Autodesk Inventor part; units mm, degrees
ref_plane "YZ Plane" through (0, 0, 0) normal (1, 0, 0) x (0, 1, 0)
ref_plane "XZ Plane" through (0, 0, 0) normal (0, 1, 0) x (-1, 0, 0)
ref_plane "XY Plane" through (0, 0, 0) normal (0, 0, 1) x (1, 0, 0)
sketch "Szkic1" plane through (0, 0, 0) normal (0, 1, 0) x (-1, 0, 0)
  line L0 (0, 10.6544) -> (0, -29.3456)
  line L1 (0, -29.3456) -> (40, -29.3456)
  line L2 (0, 10.6544) -> (40, 10.6544)
  arc A0 (40, -29.3456) -> (40, 10.6544) centre (40, -9.3456) ccw
  point P0 (0, 0)
  dimension "d0" = 40
  dimension "d1" = 40
extrude "Wyciągnięcie proste1" add sketch "Szkic1" along normal blind 9.5
sketch "Szkic2" plane through (0, 9.5, 0) normal (0, 1, 0) x (1, 0, 0)
  line L0 (-40, -10.6544) -> (0, -10.6544)
  line L1 (0.0007, -10.6544) -> (-40, -10.6544)
  arc A0 (-40, 29.3456) -> (-40, -10.6544) centre (-40, 9.3456) ccw
  circle A1 centre (-40, 9.3456) radius 15
  circle A2 centre (-40, 9.3456) radius 10
  point P0 (0, 0)
  dimension "d4" = 30
  dimension "d5" = 20
extrude "Wyciągnięcie proste2" add sketch "Szkic2" along normal blind 3
fillet "Zaokrąglenie1" radius 3 1 edges at (-55, 9.5, -9.3456)
sketch "Szkic3" plane through (0, 0, 0) normal (0, -1, 0) x (1, 0, 0)
  line L0 (0, 10.6544) -> (0, -29.3456)
  line L1 (0, -29.3456) -> (-16, -29.3456)
  line L2 (0, -29.3456) -> (-40, -29.3456)
  line L3 (-16, -29.3456) -> (-16, 10.6544)
  line L4 (-40, 10.6544) -> (0, 10.6544)
  line L5 (-16, 10.6544) -> (0, 10.6544)
  line L6 (0, 10.6544) -> (0, -29.3456)
  point P0 (0, 0)
  dimension "d9" = 16
  dimension "d10" = 40
extrude "Wyciągnięcie proste3" add sketch "Szkic3" along normal blind 12.5
sketch "Szkic4" plane through (-40, 9.5, -9.3456) normal (0, 1, 0) x (1, 0, 0)
  point P0 (40, -9.3456)
mirror "Odbij1" about plane through (-8, -12.5, -9.3456) normal (0, -1, 0)
sketch "Szkic7" plane through (0, 9.5, 10.6544) normal (1, 0, 0) x (0, 0, -1)
  point P0 (10.6544, -9.5)
sketch "Szkic8" plane through (0, 9.5, 10.6544) normal (1, 0, 0) x (0, 0, -1)
  point P0 (10.6544, -9.5)
sketch "Szkic9" plane through (0, 9.5, 10.6544) normal (1, 0, 0) x (0, 0, -1)
  line L0 (40, 0) -> (0, 0)
  line L1 (0, 0) -> (0, -22)
  line L2 (0, -44) -> (0, 0)
  line L3 (0, -22) -> (20, -22)
  circle A0 centre (20, -22) radius 16
  circle A1 centre (20, -22) radius 8
  point P0 (10.6544, -9.5)
  dimension "d15" = 22
  dimension "d16" = 32
  dimension "d17" = 16
extrude "Wyciągnięcie proste4" cut sketch "Szkic9" against normal blind 20 contours A1
sketch "Szkic10" plane through (0, 9.5, 10.6544) normal (1, 0, 0) x (0, 0, -1)
  line L0 (0, -9.5) -> (0, 0)
  line L1 (0, 0) -> (0, -22)
  line L2 (0, -22) -> (20, -22)
  circle A0 centre (20, -22) radius 16
  point P0 (10.6544, -9.5)
  dimension "d20" = 22
  dimension "d21" = 20
  dimension "d22" = 32
extrude "Wyciągnięcie proste5" add sketch "Szkic10" along normal blind 3
fillet "Zaokrąglenie2" radius 3 1 edges at (0, -12.5, 6.6544)
sketch "Szkic11" plane through (3, -12.5, -9.3456) normal (1, 0, 0) x (0, 0, -1)
  circle A0 centre (0, 0) radius 8
  point P0 (-9.3456, 12.5)
  dimension "d26" = 16
extrude "Wyciągnięcie proste6" cut sketch "Szkic11" against normal blind 20
sketch "Szkic12" plane through (0, 0, 0) normal (0, -1, 0) x (1, 0, 0)
  point P0 (0, 0)
sketch "Szkic13" plane through (-40, -34.5, -9.3456) normal (0, -1, 0) x (1, 0, 0)
  point P0 (40, 9.3456)
sketch "Szkic14" plane through (-40, 12.5, -9.3456) normal (0, 1, 0) x (1, 0, 0)
  point P0 (40, -9.3456)
sketch "Szkic15" plane through (-40, 9.5, -9.3456) normal (0, 1, 0) x (1, 0, 0)
  circle A0 centre (0, 0) radius 10
  point P0 (40, -9.3456)
  dimension "d29" = 20
extrude "Wyciągnięcie proste7" cut sketch "Szkic15" against normal blind 9.5
sketch "Szkic16" plane through (-40, -34.5, -9.3456) normal (0, -1, 0) x (1, 0, 0)
  circle A0 centre (0, 0) radius 10
  point P0 (40, 9.3456)
  dimension "d32" = 20
extrude "Wyciągnięcie proste8" cut sketch "Szkic16" against normal blind 9.5
sketch "Szkic17" plane through (0, 9.5, 0) normal (0, 1, 0) x (1, 0, 0)
  line L0 (0, -10.6544) -> (0, 29.3456)
  line L1 (0, 9.3456) -> (-10, 9.3456)
  point P0 (0, 0)
hole "Otwór1" at (-10, 9.5, -9.3456) direction (0, -1, 0) diameter 5 depth 75.75 tip angle 118
properties part number "nakrętka" material "Stal nierdzewna, austenityczna"
Work out the finished part from the listing and answer in its coordinate system (mm). A direction names the side the tool comes from. Coordinates: 2 decimals unless noted, no trailing zeros. Order: outer loops, then holes, each group sorted by start corner. A loop starts at its lowest first (then second) coordinate and runs counter-clockwise, first axis right, second up. Notation, with made-up numbers: M 35.5,21.5 L 64.5,21.5 A22 ccw 64.5,50.5 Z; hole C 37,89 d9. An arc over 180 degrees is marked long. Use CSV: the item, a comma, the result in double quotes.
1) Consider line 1 (Y direction, x = -47, z = -22.5); line 2 (Z direction, x = -40, y = -34); line 3 (Z direction, x = -3.25, y = -12.5). Determine where each line is inside the solid, lowest interval first. Write a range as [from, to].
Worked out:
line 1,"y = [-37.5, -25], [0, 12.5]"
line 2,"z = [-29.35, -19.35], [0.65, 10.65]"
line 3,"z = [-29.35, -17.35], [-1.35, 10.65]"
2) Determine the mould class of faces 4 (the face through (-16, 9.5, -9)), 5 (the face through (-6.367, -15.564, -16.736)), 6 (the face through (-15.8, -12.2, 10.654)) for opening direction Y: released by +Y, released by -Y, zero draft, split by the parting line, or undercut.
Worked out:
face 4,"released by +Y"
face 5,"undercut"
face 6,"zero draft"
3) Section A-A on x = -10 is taken. Write down the section's boundary in (y, z).
Worked out:
outline,"M -34.5,-29.35 L 9.5,-29.35 L 9.5,-11.85 L -4.9,-11.85 A8 cw -20.1,-11.85 L -34.5,-11.85 Z; M -34.5,-6.85 L -20.1,-6.85 A8 cw -4.9,-6.85 L 9.5,-6.85 L 9.5,10.65 L -34.5,10.65 Z"
4) Flat-ended cylindrical pins translate along their axes: pin 1 Ø1 at (x, z) = (-13.5, -4) entering from -Y; pin 2 Ø20 at (y, z) = (-7, -2.5) entering from -X; pin 3 Ø10 at (x, z) = (-16, -25.5) entering from +Y. Find the tip coordinate at first contact, or state that the pin passes through.
Worked out:
pin 1,"stops at y = -34.5"
pin 2,"stops at x = -60"
pin 3,"stops at y = 9.5"
5) Section C-C on z = -14.5 is taken. Count the separate pieces of the cut face and the enclosed holes in it, plus the area to 3 significant figures.
Worked out:
separate pieces,"4"
enclosed holes,"0"
area,"1,140 mm^2"
6) For faces 1 (the face through (0, 7, -9)), 2 (the face through (-28, 0, -9)), 3 (the face through (-50, -37.5, -6)), determine the directions among +Z, -Z, +X, -X, +Y, -Y from which every point of the face is accessible in a straight line to the end or side of a thin tool.
Worked out:
face 1,"+X"
face 2,"+Z, -Z, -X"
face 3,"+Z, -Z, +X, -X, -Y"
